Can you work these out from the model? Positions are in its coordinate system, mm. A direction names the side the tool comes from. Coordinates: 2 decimals unless noted, no trailing zeros. Order: outer loops, then holes, each group sorted by start corner. A loop starts at its lowest first (then second) coordinate and runs counter-clockwise, first axis right, second up. Notation, with made-up numbers: (72.25, 46.25) -> (89.25, 46.25) arc R13 ccw to (89.25, 67.25) -> close; hole circle Ø1 at (8.25, 11). An arc over 180 degrees is marked (long way). Write item = value, one per line. Start each with the question number.
from build123d import *

# Parameters (mm, degrees)
SKETCH1_W           = 25
SKETCH1_H           = 45.5
BOSS_EXTRUDE1_DEPTH = 36
BOSS_EXTRUDE2_START = -2.75
SKETCH2_W           = 36
SKETCH2_H           = 51
SKETCH2_R           = 1.5
BOSS_EXTRUDE2_DEPTH = 2
SKETCH3_R           = 11
BOSS_EXTRUDE3_DEPTH = 3.75
SKETCH4_R           = 1.5
CUT_EXTRUDE1_DEPTH  = 3.75
SKETCH5_R           = 4.25
BOSS_EXTRUDE4_DEPTH = 5.5


with BuildPart() as part:
    # Sketch1 → Boss-Extrude1 (new body)
    with BuildSketch(Plane.XY):
        Rectangle(SKETCH1_W, SKETCH1_H)
    extrude(amount=BOSS_EXTRUDE1_DEPTH)

    # Sketch2 → Boss-Extrude2 (add)
    with BuildSketch(Plane(origin=(0, 0, 0), x_dir=(-1, 0, 0), z_dir=(0, 0, -1)).offset(BOSS_EXTRUDE2_START)):
        with Locations((0, -2.75)):
            Rectangle(SKETCH2_W, SKETCH2_H)
        with Locations((-15.25, 15.25)):
            Circle(SKETCH2_R, mode=Mode.SUBTRACT)
        with Locations((-15.25, -2.25)):
            Circle(SKETCH2_R, mode=Mode.SUBTRACT)
        with Locations((-15.25, -19.25)):
            Circle(SKETCH2_R, mode=Mode.SUBTRACT)
        with Locations((-7.5, -25.5)):
            Circle(SKETCH2_R, mode=Mode.SUBTRACT)
        with Locations((7.5, -25.5)):
            Circle(SKETCH2_R, mode=Mode.SUBTRACT)
        with Locations((15.25, -19.25)):
            Circle(SKETCH2_R, mode=Mode.SUBTRACT)
        with Locations((15.25, -2.25)):
            Circle(SKETCH2_R, mode=Mode.SUBTRACT)
        with Locations((15.25, 15.25)):
            Circle(SKETCH2_R, mode=Mode.SUBTRACT)
    extrude(amount=-BOSS_EXTRUDE2_DEPTH)

    # Sketch3 → Boss-Extrude3 (add)
    with BuildSketch(Plane(origin=(0, 0, 0), x_dir=(-1, 0, 0), z_dir=(0, 0, -1))):
        with Locations((0, 10.75)):
            Circle(SKETCH3_R)
    extrude(amount=BOSS_EXTRUDE3_DEPTH)

    # Sketch4 → Cut-Extrude1 (cut)
    with BuildSketch(Plane(origin=(0, 0, -3.75), x_dir=(-1, 0, 0), z_dir=(0, 0, -1))):
        with Locations((0, 18.75)):
            Circle(SKETCH4_R)
        with Locations((-5.656854249, 16.406854249)):
            Circle(SKETCH4_R)
        with Locations((-8, 10.75)):
            Circle(SKETCH4_R)
        with Locations((-5.656854249, 5.093145751)):
            Circle(SKETCH4_R)
        with Locations((0, 2.75)):
            Circle(SKETCH4_R)
        with Locations((5.656854249, 5.093145751)):
            Circle(SKETCH4_R)
        with Locations((8, 10.75)):
            Circle(SKETCH4_R)
        with Locations((5.656854249, 16.406854249)):
            Circle(SKETCH4_R)
    extrude(amount=-CUT_EXTRUDE1_DEPTH, mode=Mode.SUBTRACT)

    # Sketch5 → Boss-Extrude4 (add)
    with BuildSketch(Plane(origin=(0, 0, -3.75), x_dir=(-1, 0, 0), z_dir=(0, 0, -1))):
        with Locations((0, 10.75)):
            Circle(SKETCH5_R)
    extrude(amount=BOSS_EXTRUDE4_DEPTH)


solid = part.part
(1) Imagine slicing it at C-C (x = -8). Write out the boundary of the cut face in (y, z).
(2) Thinking about a two-plate mould opening in X: for faces 1 (the face through (16.75, -2.18, 3.74)), 2 (the face through (-18, -3, 4)), 3 (the face through (0, -5, 0)), 4 (the face through (-6, 16, 0)), which applies, +X half, -X half, draft (parallel to the pull), parting line (faces both ways), or undercut?
(3) For faces 5 (the face through (0.195, 20.237, -1.901)), 6 (the face through (0, -22.75, 1)), 7 (the face through (0, -22.75, 20)), which set-ups out of +Z, -Z, +X, -X, +Y, -Y let a thin tool reach every point of the face, with its end or its side?
(4) Imagine slicing it at A-A (x = -15.25). Write out the boundary of the cut face in (y, z), plus the area to 3 significant figures.
(5) Imagine slicing it at B-B (y = -10.5). Write out the boundary of the cut face in (x, z), plus the area to 3 significant figures.
(6) Imagine slicing it at D-D (z = 5.5). Write out the boundary of the cut face in (x, y), plus the area to 3 significant figures.
(7) For P1, Ø1.8, axis at x = 15.25, y = 15.25, coming from the +Z side; P2, Ø2, axis at x = 3, y = -11.5, coming from the -Z side; P3, Ø4, axis at y = -9, z = 13.5, coming from the +X side; P4, Ø3.5, axis at x = 0, y = 18.75, coming from the -Z side, each with a flat end and sliding along its axis, tell me the tip position at first contact or that it passes through.
(8) If I drill on L1, parallel to Y at x = -15.25, z = 4.1; L2, parallel to X at y = -19, z = 3; L3, parallel to Y at x = -7, z = -3, over which ranges is the centre line in solid material (lowest first)? Write a range as from..to.
Result set:
q1.outline = (-28.25, 2.75) -> (-26.91, 2.75) -> (-26.91, 4.75) -> (-28.25, 4.75) -> close; (-24.09, 2.75) -> (-22.75, 2.75) -> (-22.75, 0) -> (3.2, 0) -> (3.2, -3.75) -> (9.25, -3.75) -> (9.25, 0) -> (12.25, 0) -> (12.25, -3.75) -> (18.3, -3.75) -> (18.3, 0) -> (22.75, 0) -> (22.75, 36) -> (-22.75, 36) -> (-22.75, 4.75) -> (-24.09, 4.75) -> close
q2.face_1 = undercut
q2.face_2 = -X half
q2.face_3 = draft
q2.face_4 = undercut
q3.face_5 = -Z
q3.face_6 = -Z, +X, -X, -Y
q3.face_7 = +Z, +X, -X, -Y
q4.outline = (-28.25, 2.75) -> (-20.75, 2.75) -> (-20.75, 4.75) -> (-28.25, 4.75) -> close; (-17.75, 2.75) -> (-3.75, 2.75) -> (-3.75, 4.75) -> (-17.75, 4.75) -> close; (-0.75, 2.75) -> (13.75, 2.75) -> (13.75, 4.75) -> (-0.75, 4.75) -> close; (16.75, 2.75) -> (22.75, 2.75) -> (22.75, 4.75) -> (16.75, 4.75) -> close
q4.area = 84.0 mm2
q5.outline = (-18, 2.75) -> (-12.5, 2.75) -> (-12.5, 0) -> (12.5, 0) -> (12.5, 2.75) -> (18, 2.75) -> (18, 4.75) -> (12.5, 4.75) -> (12.5, 36) -> (-12.5, 36) -> (-12.5, 4.75) -> (-18, 4.75) -> close
q5.area = 922 mm2
q6.outline = (-12.5, -22.75) -> (12.5, -22.75) -> (12.5, 22.75) -> (-12.5, 22.75) -> close
q6.area = 1,140 mm2
q7.P1 = through
q7.P2 = 0
q7.P3 = 12.5
q7.P4 = -3.75
q8.L1 = -28.25..-20.75, -17.75..-3.75, -0.75..13.75, 16.75..22.75
q8.L2 = -18..-16.73, -13.77..13.77, 16.73..18
q8.L3 = 2.26..4.43, 5.76..9.63, 11.87..15.74, 17.07..19.24
